For this review, take the finished solid that the model builds, in its own axes (mm). Coordinates: 2 decimals unless noted, no trailing zeros. Write each loop counter-clockwise with the first axis right and the second up, starting at its lowest first coordinate (ties: lowest second). Pieces come first, ordered by that corner, then holes.
Autodesk Inventor part; units mm, degrees
ref_plane "YZ Plane" through (0, 0, 0) normal (1, 0, 0) x (0, 1, 0)
ref_plane "XZ Plane" through (0, 0, 0) normal (0, 1, 0) x (-1, 0, 0)
ref_plane "XY Plane" through (0, 0, 0) normal (0, 0, 1) x (1, 0, 0)
sketch "스케치1" plane through (0, 0, 0) normal (0, 1, 0) x (-1, 0, 0)
  line L0 (60, -100) -> (-60, -100)
  line L1 (-60, -100) -> (-60, 100)
  line L2 (-60, 100) -> (60, 100)
  line L3 (60, 100) -> (60, -100)
  line L4 (60, -100) -> (-60, 100) construction
  line L5 (-60, -100) -> (60, 100) construction
  point P0 (0, 0)
  dimension "d0" = 200
  dimension "d1" = 120
extrude "돌출1" add sketch "스케치1" along normal blind 3
sketch "스케치3" plane through (0, 3, 0) normal (0, 1, 0) x (1, 0, 0)
  line L0 (-43.6, -60) -> (25, -60)
  line L1 (25, -60) -> (25, -6.6)
  line L2 (25, -6.6) -> (-43.6, -6.6)
  line L3 (-43.6, -6.6) -> (-43.6, -60)
  circle A0 centre (9.7, -57.45) radius 1.6
  circle A1 centre (11.03, -9.15) radius 1.6
  circle A2 centre (-41.05, -42.16) radius 1.6
  circle A3 centre (-41.05, -14.23) radius 1.6
  line L4 (60, -100) -> (60, 100)
  line L5 (-60, -100) -> (60, -100)
  point P0 (0, 0)
  point P1 (0, 0)
  dimension "d22" = 68.6
  dimension "d23" = 53.4
  dimension "d26" = 3.2
  dimension "d27" = 15.3
  dimension "d28" = 2.55
  dimension "d29" = 3.2
  dimension "d30" = 13.97
  dimension "d31" = 2.55
  dimension "d32" = 3.2
  dimension "d33" = 35.56
  dimension "d34" = 3.2
  dimension "d35" = 2.55
  dimension "d36" = 2.55
  dimension "d37" = 7.63
  dimension "d38" = 35
  dimension "d40" = 40
extrude "돌출2" cut sketch "스케치3" against normal through all contours A0 | A1 | A2 | A3
sketch "스케치4" plane through (0, 3, 0) normal (0, 1, 0) x (1, 0, 0)
  line L0 (5, 15) -> (45, 15)
  line L1 (45, 15) -> (45, 55)
  line L2 (45, 55) -> (5, 55)
  line L3 (5, 55) -> (5, 15)
  circle A0 centre (5, 15) radius 1.6
  circle A1 centre (5, 55) radius 1.6
  circle A2 centre (45, 55) radius 1.6
  circle A3 centre (45, 15) radius 1.6
  line L4 (-47.9371, 14.7215) -> (-7.9371, 14.7215)
  line L5 (-7.9371, 14.7215) -> (-7.9371, 64.7215)
  line L6 (-7.9371, 64.7215) -> (-47.9371, 64.7215)
  line L7 (-47.9371, 64.7215) -> (-47.9371, 14.7215)
  line L8 (60, -100) -> (60, 100)
  line L9 (60, 100) -> (-60, 100)
  circle A4 centre (-15, -1) radius 10
  line L10 (-60, 100) -> (-60, -100)
  point P0 (0, 0)
  point P1 (0, 0)
  dimension "d43" = 40
  dimension "d44" = 40
  dimension "d47" = 3.2
  dimension "d48" = 3.2
  dimension "d49" = 3.2
  dimension "d50" = 3.2
  dimension "d51" = 40
  dimension "d52" = 50
  dimension "d53" = 15
  dimension "d54" = 45
  dimension "d56" = 20
  dimension "d69" = 45
  dimension "d70" = 101
extrude "돌출3" cut sketch "스케치4" against normal through all contours L3 A0 L0 | L0 A0 L3 | A3 L1 L0 | L0 L1 A3 | A1 L2 L3 | L3 L2 A1 | A2 L2 L1 | L1 L2 A2 | A4
sketch "스케치5" plane through (0, 3, 0) normal (0, 1, 0) x (1, 0, 0)
  line L0 (57, -25) -> (61.988, -25)
  line L1 (61.988, -25) -> (61.988, 25)
  line L2 (61.988, 25) -> (57, 25)
  line L3 (57, 25) -> (57, -25)
  line L4 (60, -100) -> (60, 100)
  line L5 (60, 100) -> (-60, 100)
  line L6 (0, -100) -> (0, 100)
  line L7 (60, 100) -> (-60, 100)
  line L8 (-57, -25) -> (-61.988, -25)
  line L9 (-61.988, -25) -> (-61.988, 25)
  line L10 (-61.988, 25) -> (-57, 25)
  line L11 (-57, 25) -> (-57, -25)
  point P0 (0, 0)
  dimension "d59" = 50
  dimension "d60" = 3
  dimension "d61" = 75
extrude "돌출4" cut sketch "스케치5" against normal through all
sketch "스케치6" plane through (0, 3, 0) normal (0, 1, 0) x (1, 0, 0)
  line L0 (-15, -110.8891) -> (15, -110.8891)
  line L1 (15, -110.8891) -> (15, -97)
  line L2 (15, -97) -> (-15, -97)
  line L3 (-15, -97) -> (-15, -110.8891)
  line L4 (-60, -100) -> (60, -100)
  line L5 (-60, -25) -> (-60, -100)
  line L6 (-57, -25) -> (-57, 25)
  line L7 (-57, 0) -> (56.7319, 0)
  line L8 (-15, 110.8891) -> (15, 110.8891)
  line L9 (15, 110.8891) -> (15, 97)
  line L10 (15, 97) -> (-15, 97)
  line L11 (-15, 97) -> (-15, 110.8891)
  point P0 (0, 0)
  dimension "d64" = 30
  dimension "d65" = 3
  dimension "d66" = 45
extrude "돌출5" cut sketch "스케치6" against normal through all
sketch "스케치7" plane through (0, 3, 0) normal (0, 1, 0) x (1, 0, 0)
  point P0 (0, 0)
sketch "스케치9" plane through (0, 3, 0) normal (0, 1, 0) x (1, 0, 0)
  circle A0 centre (-43, -75) radius 1.6
  circle A1 centre (-43, -67) radius 1.6
  line L0 (-60, -25) -> (-60, -100)
  line L1 (-60, -100) -> (-15, -100)
  line L2 (-15, -97) -> (15, -97)
  line L3 (0, -97) -> (0, 96.8174)
  line L4 (-57, -25) -> (-57, 25)
  line L5 (-57, 0) -> (57, 0)
  line L6 (57, 25) -> (57, -25)
  circle A2 centre (-43, 75) radius 1.6
  circle A3 centre (-43, 67) radius 1.6
  circle A4 centre (43, -75) radius 1.6
  circle A5 centre (43, -67) radius 1.6
  circle A6 centre (43, 75) radius 1.6
  circle A7 centre (43, 67) radius 1.6
  point P0 (0, 0)
  dimension "d75" = 3.2
  dimension "d76" = 3.2
  dimension "d77" = 8
  dimension "d78" = 17
  dimension "d79" = 17
  dimension "d80" = 25
extrude "돌출7" cut sketch "스케치9" against normal through all
properties part number "본체 밑판 레이저 수정"
1) Consider section A-A (y = 0.7). Count the separate pieces of the cut face and the enclosed holes in it, then the cut area to 3 significant figures.
2) Clearance check with flat-ended pins moving along their axes: P1, Ø3.5, axis at x = 43, z = -75, coming from the -Y side; P2, Ø1.5, axis at y = 1.5, z = -7.5, coming from the -X side. State where each tip first meets the part, or that it passes through.
3) Consider section B-B (x = 1). Give the boundary of the cut face in (y, z), then the cut area to 3 significant figures.
4) For L1, parallel to Z at x = 43, y = 0.75; L2, parallel to X at y = 1.15, z = -15; L3, parallel to Z at x = -41.05, y = 1.2, list the stretches that pass through material, from the lowest coordinate up.
5) The part is to be moulded in two halves that separate along Z. For faces 1 (the face through (-5.763, 1.521, 4.83)), 2 (the face through (1, 0, 1)), say which applies: pulls with the +Z half, pulls with the -Z half, needs draft (parallel to the pull), parting line crosses it, or undercut.
Results:
1. separate pieces: 1
1. enclosed holes: 17
1. area: 23,100 mm2
2. P1: stops at y = 0
2. P2: stops at x = -57
3. outline: (0, -97) - (3, -97) - (3, 97) - (0, 97) - close
3. area: 582 mm2
4. L1: z = -100 to -76.6, -73.4 to -68.6, -65.4 to 65.4, 68.6 to 73.4, 76.6 to 100
4. L2: x = -57 to 3.4, 6.6 to 43.4, 46.6 to 57
4. L3: z = -100 to 12.63, 15.83 to 40.56, 43.76 to 100
5. face 1: undercut
5. face 2: needs draft
